from build123d import *

# Parameters (mm, degrees)
CROQUIS5_R            = 1.9
CORTAR_EXTRUIR1_DEPTH = 50.497474683
MATRIZC1_COUNT        = 3


with BuildPart() as part:
    # Croquis4 → Revolución1 (revolve)
    with BuildSketch(Plane(origin=(0, 0, 0), x_dir=(0, 0, -1), z_dir=(1, 0, 0))):
        Polygon((-15, 0), (0, 0), (0, 1), (-14.585786438, 1), (-33.585786438, 20), (-35, 20), align=None)
    revolve(axis=Axis((0, 0, 0), (0, 1, 0)))

    # Croquis5 → Cortar-Extruir1 (cut, through all)
    with BuildSketch(Plane(origin=(-7.5, -7.5, -10.606601718), x_dir=(0.5, -0.5, -0.707106781), z_dir=(0.707106781, 0.707106781, 0))):
        with Locations((-25, 10.353571071)):
            Circle(CROQUIS5_R)
    cortar_extruir1 = extrude(amount=CORTAR_EXTRUIR1_DEPTH, mode=Mode.SUBTRACT)

    # MatrizC1: Cortar-Extruir1 ×3 about axis
    matrizc1_axis = Axis((0, 1, 0), (0, 1, 0))
    for i in range(1, MATRIZC1_COUNT):
        add(cortar_extruir1.rotate(matrizc1_axis, i * 360 / MATRIZC1_COUNT), mode=Mode.SUBTRACT)


solid = part.part
Source: CAD feature listing. Evaluate the final solid. Frame: model axes, mm. A direction names the side the tool comes from. Coordinates: 2 decimals unless noted, no trailing zeros. Order: outer loops, then holes, each group sorted by start corner. A loop starts at its lowest first (then second) coordinate and runs counter-clockwise, first axis right, second up.
Item 1: Material intervals for line 1 (X direction, y = 18.25, z = -15); line 2 (Z direction, x = 3.5, y = 1.75); line 3 (X direction, y = 10, z = 8), sorted ascending.
Output values:
line 1: x = -29.67 to -28.08, 28.08 to 29.67
line 2: z = -16.38 to -14.93, 14.93 to 16.38
line 3: x = -23.69 to -22.19, 22.19 to 23.69
Item 2: First-contact query: P1, Ø4, axis at y = 17.5, z = -18, coming from the -X side; P2, Ø1.5, axis at y = 7.5, z = 19, coming from the -X side; P3, Ø14.5, axis at x = -1.5, z = -4, coming from the +Y side. Flat tips, straight axial feed; report the tip coordinate or a pass-through.
Output values:
P1: stops at x = -29.72
P2: stops at x = -13.77
P3: stops at y = 1
Item 3: Cut plane D-D (y = 16.75). Return loops of the section in (x, z).
Output values:
outline: circle Ø63.5 at (0, 0); hole circle Ø60.67 at (0, 0)
Item 4: Cut plane A-A (z = 0). Return loops of the section in (x, y), plus the area to 3 significant figures.
Output values:
outline: (-35, 20) - (-26.51, 11.51) - (-25.8, 12.22) - (-33.59, 20) - close; (-23.84, 8.84) - (-15, 0) - (15, 0) - (35, 20) - (33.59, 20) - (14.59, 1) - (-14.59, 1) - (-23.14, 9.55) - close
area: 81.0 mm2
Item 5: Cut plane C-C (y = 4). Return loops of the section in (x, z).
Output values:
outline: circle Ø38 at (0, 0); hole circle Ø35.17 at (0, 0)
Item 6: Set-up query: faces 1 (the face through (13.9, 10.7, 20.8)), 2 (the face through (0, 1, 0)). Return all of +Z, -Z, +X, -X, +Y, -Y with unobstructed straight access to the full face (end or side cutting, diameter ignored); none if empty.
Output values:
face 1: none
face 2: +Y
Item 7: Pull-direction query (Z, two-part tool) for faces 3 (the face through (-24.981, 10.725, 1.634)), 4 (the face through (11.076, 10.725, -22.451)), 5 (the face through (4.8, 0.97, 15.23)), 6 (the face through (13.1, 20, 31.3)); classes: pulls with the +Z half, pulls with the -Z half, needs draft (parallel to the pull), parting line crosses it, or undercut.
Output values:
face 3: undercut
face 4: undercut
face 5: parting line crosses it
face 6: needs draft
Item 8: Cut plane B-B (x = 0). Return loops of the section in (y, z), plus the area to 3 significant figures.
Output values:
outline: (0, -15) - (20, -35) - (20, -33.59) - (1, -14.59) - (1, 14.59) - (20, 33.59) - (20, 35) - (0, 15) - close
area: 84.7 mm2
